```python
from build123d import *

# Parameters (mm, degrees)
SKETCH1_W                     = 199.9
SKETCH1_H                     = 95
BOSS_EXTRUDE1_DEPTH           = 5
CBORE_FOR_M4_SHCS1_AT_2_COUNT = 2
CBORE_FOR_M4_SHCS1_AT_2_PITCH = 69.462381906
CBORE_FOR_M4_SHCS1_AT_3_COUNT = 2
CBORE_FOR_M4_SHCS1_AT_3_PITCH = 162.557751276
CBORE_FOR_M4_SHCS1_AT_4_COUNT = 2
CBORE_FOR_M4_SHCS1_AT_4_PITCH = 27.5
F_6_1_6_1_DIAMETER_HOLE2_D    = 6.1
LPATTERN1_COUNT               = 2
LPATTERN1_PITCH               = 35
SKETCH6_W                     = 41
SKETCH6_H                     = 40
CUT_EXTRUDE1_DEPTH            = 6
LPATTERN2_COUNT               = 2
LPATTERN2_PITCH               = 65
FILLET1_R                     = 5
F_6_1_6_1_DIAMETER_HOLE1_D    = 6.1


with BuildPart() as part:
    # Sketch1 → Boss-Extrude1 (new body)
    with BuildSketch(Plane(origin=(0, 0, 0), x_dir=(1, 0, 0), z_dir=(0, 1, 0))):
        with Locations((99.95, -47.5)):
            Rectangle(SKETCH1_W, SKETCH1_H)
    extrude(amount=BOSS_EXTRUDE1_DEPTH)

    # Sketch3 → CBORE for M4 SHCS1 (revolve, cut)
    with BuildSketch(Plane(origin=(179.9, 0, 15.15), x_dir=(0, 0, -1), z_dir=(1, 0, 0))):
        Polygon((0, 0), (0, 5), (2.25, 5), (2.25, 4), (4, 4), (4, 0.025), (4.025, 0), align=None)
    cbore_for_m4_shcs1 = revolve(axis=Axis((179.9, -6.35, 15.15), (0, 1, 0)), mode=Mode.SUBTRACT)

    # CBORE for M4 SHCS1 at 2: CBORE for M4 SHCS1 ×2
    with Locations(*[Vector(-0.431888443, 0, 0.901927033) * (i * CBORE_FOR_M4_SHCS1_AT_2_PITCH) for i in range(1, CBORE_FOR_M4_SHCS1_AT_2_COUNT)]):
        add(cbore_for_m4_shcs1, mode=Mode.SUBTRACT)

    # CBORE for M4 SHCS1 at 3: CBORE for M4 SHCS1 ×2
    with Locations(*[Vector(-0.922748985, 0, 0.385401493) * (i * CBORE_FOR_M4_SHCS1_AT_3_PITCH) for i in range(1, CBORE_FOR_M4_SHCS1_AT_3_COUNT)]):
        add(cbore_for_m4_shcs1, mode=Mode.SUBTRACT)

    # CBORE for M4 SHCS1 at 4: CBORE for M4 SHCS1 ×2
    with Locations(*[(0, 0, i * CBORE_FOR_M4_SHCS1_AT_4_PITCH) for i in range(1, CBORE_FOR_M4_SHCS1_AT_4_COUNT)]):
        add(cbore_for_m4_shcs1, mode=Mode.SUBTRACT)

    # Ø6.1 (6.1) Diameter Hole2 (through all)
    with Locations(Plane(origin=(0, 5, 0), x_dir=(1, 0, 0), z_dir=(0, 1, 0))):
        with Locations((170, -15), (20, -15), (50, -15), (80, -15), (110, -15), (140, -15)):
            f_6_1_6_1_diameter_hole2 = Hole(F_6_1_6_1_DIAMETER_HOLE2_D / 2)

    # LPattern1: Ø6.1 (6.1) Diameter Hole2 ×2
    with Locations(*[(0, 0, i * LPATTERN1_PITCH) for i in range(1, LPATTERN1_COUNT)]):
        add(f_6_1_6_1_diameter_hole2, mode=Mode.SUBTRACT)

    # Sketch6 → Cut-Extrude1 (cut, through all)
    with BuildSketch(Plane(origin=(0, 5, 0), x_dir=(1, 0, 0), z_dir=(0, 1, 0))):
        with Locations((179.4, -75)):
            Rectangle(SKETCH6_W, SKETCH6_H)
    extrude(amount=-CUT_EXTRUDE1_DEPTH, mode=Mode.SUBTRACT)

    # LPattern2: Ø6.1 (6.1) Diameter Hole2 ×2
    with Locations(*[(0, 0, i * LPATTERN2_PITCH) for i in range(1, LPATTERN2_COUNT)]):
        add(f_6_1_6_1_diameter_hole2, mode=Mode.SUBTRACT)

    # Fillet1
    fillet1_edges = [part.edges().sort_by_distance(p)[0] for p in [
        (199.9, 2.5, 55),
        (158.9, 2.5, 95),
        (158.9, 2.5, 55),
        (0, 2.5, 0),
        (0, 2.5, 95),
    ]]
    fillet(fillet1_edges, radius=FILLET1_R)

    # Ø6.1 (6.1) Diameter Hole1 (through all)
    with Locations(Plane(origin=(0, 5, 0), x_dir=(1, 0, 0), z_dir=(0, 1, 0))):
        with Locations((192, -50), (192, -7.5)):
            Hole(F_6_1_6_1_DIAMETER_HOLE1_D / 2)


solid = part.part
```
Can you work these out from the model? Positions are in its coordinate system, mm. A direction names the side the tool comes from. Coordinates: 2 decimals unless noted, no trailing zeros. Write each loop counter-clockwise with the first axis right and the second up, starting at its lowest first coordinate (ties: lowest second). Pieces come first, ordered by that corner, then holes. Notation, with made-up numbers: M -34.5,53 L -24.5,53 A26 cw -24.5,82 Z; hole C -16.5,35.25 d11. An arc over 180 degrees is marked long. Write item = value, one per line. Start each with the question number.
Q1. Thinking about a two-plate mould opening in Z: for faces 3 (the face through (0, 2, 48)), 4 (the face through (83.047, 2.465, 14.866)), 5 (the face through (32, 4, 80)), 6 (the face through (179, 3, 55)), which applies, released by +Z, released by -Z, zero draft, split by the parting line, or undercut?
Q2. I'm going to push flat-ended pins straight in: pin 1 (1.5 mm diameter, centred on x = 177.5, y = 1, fed in from +Z); pin 2 (10 mm diameter, centred on x = 80, z = 50, fed in from -Y); pin 3 (5 mm diameter, centred on x = 80, z = 80, fed in from -Y); pin 4 (7 mm diameter, centred on x = 179.9, z = 42.65, fed in from -Y). Where does each tip first touch, or does it pass through?
Q3. If we section it at A-A, the plane x = 179.9: Write out the boundary of the cut face in (y, z) (3 decimals).
Q4. If I drill on L1, parallel to Z at x = 50, y = 3.7; L2, parallel to X at y = 1.2, z = 76; L3, parallel to Z at x = 19, y = 4.3, over which ranges is the centre line in solid material (lowest first)? Write a range as [from, to].
Q5. If we section it at B-B, the plane z = 7.5: Write out the boundary of the cut face in (x, y).
Q6. On a 3-axis mill with a long thin cutter (end or side, diameter ignored), from which of +Z, -Z, +X, -X, +Y, -Y can I reach the whole of each face in a straight line? I mean faces 1 (the face through (30.76, 4.49, 75.72)), 2 (the face through (182, 4, 17)). Say none if no direction works.
Q7. If we section it at C-C, the plane y = 1.9: State how many separate pieces and enclosed holes the cut face has, then the cut area to 3 significant figures.
Q8. If we section it at D-D, the plane x = 140: Write out the boundary of the cut face in (y, z).
Check sheet entries:
q1.face_3 = zero draft
q1.face_4 = undercut
q1.face_5 = undercut
q1.face_6 = released by +Z
q2.pin_1 = 55
q2.pin_2 = 0
q2.pin_3 = through
q2.pin_4 = 4
q3.outline = M 0,0 L 5,0 L 5,12.9 L 4,12.9 L 4,11.15 L 0.025,11.15 L 0,11.125 Z; M 0,19.175 L 0.025,19.15 L 4,19.15 L 4,17.4 L 5,17.4 L 5,40.4 L 4,40.4 L 4,38.65 L 0.025,38.65 L 0,38.625 Z; M 0,46.675 L 0.025,46.65 L 4,46.65 L 4,44.9 L 5,44.9 L 5,55 L 0,55 Z
q4.L1 = [0, 11.95], [18.05, 46.95], [53.05, 76.95], [83.05, 95]
q4.L2 = [0, 26.33], [33.47, 146.33], [153.47, 158.9]
q4.L3 = [0, 12.12], [17.88, 47.12], [52.88, 77.12], [82.88, 95]
q5.outline = M 0,0 L 188.95,0 L 188.95,5 L 0,5 Z; M 195.05,0 L 199.9,0 L 199.9,5 L 195.05,5 Z
q6.face_1 = +Y, -Y
q6.face_2 = -Y
q7.separate_pieces = 1
q7.enclosed_holes = 23
q7.area = 16,600 mm²
q8.outline = M 0,0 L 5,0 L 5,11.95 L 0,11.95 Z; M 0,18.05 L 5,18.05 L 5,46.95 L 0,46.95 Z; M 0,53.05 L 5,53.05 L 5,76.95 L 0,76.95 Z; M 0,83.05 L 5,83.05 L 5,95 L 0,95 Z
